Geometry check sheet. Reference: the model listing, model coordinates, mm. A direction names the side the tool comes from. Round coordinates to 2 decimals unless told otherwise and drop trailing zeros. Write each loop counter-clockwise with the first axis right and the second up, starting at its lowest first coordinate (ties: lowest second). Pieces come first, ordered by that corner, then holes. Notation, with made-up numbers: (1.25, -4.75) - (56.25, -4.75) arc R15 ccw to (56.25, 19.25) - close; hole circle Ø10 at (52, -1.5). An arc over 180 degrees is marked (long way). Return JSON: item names as keys, results as strings.
```python
from build123d import *

# Parameters (mm, degrees)
SKETCH1_W           = 43.2816
SKETCH1_H           = 21.1074
BOSS_EXTRUDE1_DEPTH = 1.651
SKETCH2_R           = 1.4732
CUT_EXTRUDE1_DEPTH  = 49.18241416
SKETCH3_R           = 3.9878
BOSS_EXTRUDE2_DEPTH = 10.668
SKETCH4_W           = 10.16
SKETCH4_H           = 8.382
BOSS_EXTRUDE3_DEPTH = 3.7338
SKETCH4_3_W         = 11.684
SKETCH4_3_H         = 11.684
BOSS_EXTRUDE4_DEPTH = 7.62
SKETCH4_4_W         = 9.5758
SKETCH4_4_H         = 4.7498
BOSS_EXTRUDE5_DEPTH = 9.652
SKETCH5_R           = 1.016
BOSS_EXTRUDE6_DEPTH = 0.762
SKETCH6_W           = 4.064
SKETCH6_H           = 4.064
BOSS_EXTRUDE7_DEPTH = 0.1524
SKETCH7_R           = 0.381
CUT_EXTRUDE2_DEPTH  = 50.288914339


with BuildPart() as part:
    # Sketch1 → Boss-Extrude1 (new body)
    with BuildSketch(Plane.XY):
        with Locations((21.6408, 10.5537)):
            Rectangle(SKETCH1_W, SKETCH1_H)
    extrude(amount=BOSS_EXTRUDE1_DEPTH)

    # Sketch2 → Cut-Extrude1 (cut, through all)
    with BuildSketch(Plane.XY.offset(1.651)):
        with Locations((36.6268, 18.4658)):
            Circle(SKETCH2_R)
        with Locations((6.7564, 2.6416)):
            Circle(SKETCH2_R)
    extrude(amount=-CUT_EXTRUDE1_DEPTH, mode=Mode.SUBTRACT)

    # Sketch3 → Boss-Extrude2 (add)
    with BuildSketch(Plane(origin=(0, 0, 0), x_dir=(-1, 0, 0), z_dir=(0, 0, -1))):
        with Locations((-4.5593, 10.5537)):
            Circle(SKETCH3_R)
        with Locations((-38.7223, 10.5537)):
            Circle(SKETCH3_R)
    extrude(amount=BOSS_EXTRUDE2_DEPTH)

    # Sketch4 → Boss-Extrude3 (add)
    with BuildSketch(Plane(origin=(0, 0, 0), x_dir=(-1, 0, 0), z_dir=(0, 0, -1))):
        with Locations((-28.0416, 14.3764)):
            Rectangle(SKETCH4_W, SKETCH4_H)
    extrude(amount=BOSS_EXTRUDE3_DEPTH)

    # Sketch4_3 → Boss-Extrude4 (add)
    with BuildSketch(Plane(origin=(0, 0, 0), x_dir=(-1, 0, 0), z_dir=(0, 0, -1))):
        with Locations((-15.494, 7.112)):
            Rectangle(SKETCH4_3_W, SKETCH4_3_H)
    extrude(amount=BOSS_EXTRUDE4_DEPTH)

    # Sketch4_4 → Boss-Extrude5 (add)
    with BuildSketch(Plane(origin=(0, 0, 0), x_dir=(-1, 0, 0), z_dir=(0, 0, -1))):
        with Locations((-14.9479, 17.4625)):
            Rectangle(SKETCH4_4_W, SKETCH4_4_H)
    extrude(amount=BOSS_EXTRUDE5_DEPTH)

    # Sketch5 → Boss-Extrude6 (add)
    with BuildSketch(Plane(origin=(0, 0, -9.652), x_dir=(-1, 0, 0), z_dir=(0, 0, -1))):
        with Locations(Location((-17.9578, 18.3134, 0), (0, 0, 180))):
            Circle(SKETCH5_R)
    extrude(amount=BOSS_EXTRUDE6_DEPTH)

    # Sketch6 → Boss-Extrude7 (add)
    with BuildSketch(Plane(origin=(0, 0, 0), x_dir=(-1, 0, 0), z_dir=(0, 0, -1))):
        with Locations((-41.2496, 19.0754)):
            Rectangle(SKETCH6_W, SKETCH6_H)
        with Locations((-41.2496, 2.032)):
            Rectangle(SKETCH6_W, SKETCH6_H)
        with Locations((-2.032, 19.0754)):
            Rectangle(SKETCH6_W, SKETCH6_H)
        with Locations((-2.032, 2.032)):
            Rectangle(SKETCH6_W, SKETCH6_H)
    extrude(amount=BOSS_EXTRUDE7_DEPTH)

    # Sketch7 → Cut-Extrude2 (cut, through all)
    with BuildSketch(Plane(origin=(0, 0, -0.1524), x_dir=(-1, 0, 0), z_dir=(0, 0, -1))):
        with Locations((-41.2496, 19.0754)):
            Circle(SKETCH7_R)
        with Locations(Location((-2.032, 19.0754, 0), (0, 0, 180))):
            Circle(SKETCH7_R)
        with Locations((-2.032, 2.032)):
            Circle(SKETCH7_R)
        with Locations(Location((-41.2496, 2.032, 0), (0, 0, 180))):
            Circle(SKETCH7_R)
    extrude(amount=-CUT_EXTRUDE2_DEPTH, mode=Mode.SUBTRACT)


solid = part.part
```
(1) Access from +Z, -Z, +X, -X, +Y, -Y to the whole of each face (thin tool, end or side, straight path). Record for faces 4 (the face through (34.92, 11.75, -5.26)), 5 (the face through (41, 20, -0.152)), 6 (the face through (9.652, 7, -4)).
Response values:
{"face 4": "-Z", "face 5": "-Z, +X, +Y", "face 6": "-Z, +Y, -Y"}
(2) Release check for a two-part mould opening along X. For faces 1 (the face through (28, 10.185, -2)), 2 (the face through (18.927, 18.008, -10.028)), 3 (the face through (15, 17, -9.652)) record: pulls with the +X half, pulls with the -X half, needs draft (parallel to the pull), parting line crosses it, or undercut.
Response values:
{"face 1": "undercut", "face 2": "parting line crosses it", "face 3": "needs draft"}
(3) Gauge pin test, flat ends, axial feed: pin 1 (5 mm diameter, centred on x = 14, y = 18, fed in from -Z); pin 2 (3.5 mm diameter, centred on x = 41, y = 18.5, fed in from -Z); pin 3 (3 mm diameter, centred on x = 27.5, z = -2, fed in from -Y). Record the tip position at first contact, or that the pin passes through.
Response values:
{"pin 1": "stops at z = -9.65", "pin 2": "stops at z = -0.15", "pin 3": "stops at y = 10.19"}
(4) Section check A-A, the plane z = -1.5. Enter the section's corners in (x, y).
Response values:
{"outline": "circle Ø7.98 at (4.56, 10.55); (9.65, 1.27) - (21.34, 1.27) - (21.34, 12.95) - (9.65, 12.95) - close; (10.16, 15.09) - (19.74, 15.09) - (19.74, 19.84) - (10.16, 19.84) - close; (22.96, 10.19) - (33.12, 10.19) - (33.12, 18.57) - (22.96, 18.57) - close; circle Ø7.98 at (38.72, 10.55)"}
(5) Section check B-B, the plane x = 37.5. Enter the section's corners in (y, z).
Response values:
{"outline": "(0, 0) - (6.76, 0) - (6.76, -10.67) - (14.35, -10.67) - (14.35, 0) - (17.28, 0) - (17.28, 1.65) - (0, 1.65) - close; (19.65, 0) - (21.11, 0) - (21.11, 1.65) - (19.65, 1.65) - close"}
(6) Section check D-D, the plane x = 16. Enter the section's corners in (y, z).
Response values:
{"outline": "(0, 0) - (1.27, 0) - (1.27, -7.62) - (12.95, -7.62) - (12.95, 0) - (15.09, 0) - (15.09, -9.65) - (19.84, -9.65) - (19.84, 0) - (21.11, 0) - (21.11, 1.65) - (0, 1.65) - close"}
(7) Material ranges on line 1 along Z through (x, y) = (15.5, 5.5); line 2 along Z through (x, y) = (39.5, 1.5); line 3 along X through (y, z) = (6.5, -1.25), recorded low to high. Write a range as [from, to].
Response values:
{"line 1": "z = [-7.62, 1.65]", "line 2": "z = [-0.15, 1.65]", "line 3": "x = [9.65, 21.34]"}
(8) Section check C-C, the plane y = 3.5. Enter the section's corners in (x, z), plus the area to 3 significant figures.
Response values:
{"outline": "(0, -0.15) - (4.06, -0.15) - (4.06, 0) - (5.56, 0) - (5.56, 1.65) - (0, 1.65) - close; (7.95, 0) - (9.65, 0) - (9.65, -7.62) - (21.34, -7.62) - (21.34, 0) - (39.22, 0) - (39.22, -0.15) - (43.28, -0.15) - (43.28, 1.65) - (7.95, 1.65) - close", "area": "158 mm^2"}
